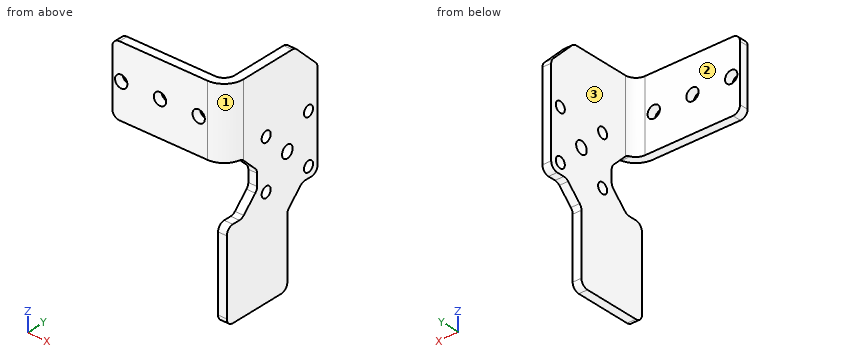
```python
from build123d import *

# Parameters (mm, degrees)
T_LE_DE_BASE_PLI_E1_DEPTH    = 40
BOSS_EXTRU_1_DEPTH           = 5
ENL_V_MAT_EXTRU_1_DEPTH      = 117.833214455
ENL_V_MAT_EXTRU_1_DEPTH_BACK = 117.833214455
ESQUISSE8_R                  = 3.5
ESQUISSE8_R_2                = 3
ESQUISSE10_W                 = 50
ESQUISSE10_H                 = 20
BOSS_EXTRU_2_DEPTH           = 5
ENL_V_MAT_EXTRU_2_DEPTH      = 117.833214455
ENL_V_MAT_EXTRU_2_DEPTH_BACK = 117.833214455
ESQUISSE9_R                  = 3.5
ENL_V_MAT_EXTRU_3_DEPTH      = 115.127122105
ENL_V_MAT_EXTRU_3_DEPTH_BACK = 115.127122105
ESQUISSE11_W                 = 50
ESQUISSE11_H                 = 20
CHANFREIN1_SIZE              = 10
CONG_1_R                     = 4


# Read off the part's stored shape, not the designer's step: Tôle de base pliée1
with BuildPart() as part:
    # Tôle de base pliée1 outline → Tôle de base pliée1 (new body)
    with BuildSketch(Plane.XY):
        with BuildLine():
            Line((65, 6), (65, 40))
            Line((65, 40), (60, 40))
            Line((60, 40), (60, 6))
            ThreePointArc((60, 6), (58.242640687, 1.757359313), (54, 0))
            Line((54, 0), (0, 0))
            Line((0, 0), (0, -5))
            Line((0, -5), (54, -5))
            ThreePointArc((54, -5), (61.778174593, -1.778174593), (65, 6))
        make_face()
    extrude(amount=T_LE_DE_BASE_PLI_E1_DEPTH)

    # Esquisse7 → Boss.-Extru.1 (add)
    with BuildSketch(Plane.ZY.offset(-60)):
        Polygon((25, 55), (-80, 55), (-80, 15), (0, 15), (40, 40), align=None)
    extrude(amount=-BOSS_EXTRU_1_DEPTH)

    # Esquisse8 → Enlèv. mat.-Extru.1 (cut, two sides: drawn at the far end of the back side and taken through both)
    with BuildSketch(Plane(origin=(65, 0, 0), x_dir=(0, 0, -1), z_dir=(1, 0, 0)).offset(-ENL_V_MAT_EXTRU_1_DEPTH_BACK)):
        with Locations(Location((10, 35, 0), (0, 0, 180))):
            Circle(ESQUISSE8_R)
        with Locations(Location((24, 49, 0), (0, 0, 180))):
            Circle(ESQUISSE8_R_2)
        with Locations(Location((24, 21, 0), (0, 0, 180))):
            Circle(ESQUISSE8_R_2)
        with Locations(Location((-4, 21, 0), (0, 0, 180))):
            Circle(ESQUISSE8_R_2)
        with Locations(Location((-4, 49, 0), (0, 0, 180))):
            Circle(ESQUISSE8_R_2)
    extrude(amount=ENL_V_MAT_EXTRU_1_DEPTH + ENL_V_MAT_EXTRU_1_DEPTH_BACK, mode=Mode.SUBTRACT)

    # Esquisse10 → Boss.-Extru.2 (add)
    with BuildSketch(Plane.ZY.offset(-60)):
        with Locations((-55, 5)):
            Rectangle(ESQUISSE10_W, ESQUISSE10_H)
    extrude(amount=-BOSS_EXTRU_2_DEPTH)

    # Esquisse9 → Enlèv. mat.-Extru.2 (cut, two sides: drawn at the far end of the back side and taken through both)
    with BuildSketch(Plane(origin=(0, 0, 0), x_dir=(1, 0, 0), z_dir=(0, 1, 0)).offset(-ENL_V_MAT_EXTRU_2_DEPTH_BACK)):
        with Locations(Location((5, -20, 0), (0, 0, 270))):
            Circle(ESQUISSE9_R)
        with Locations(Location((27, -20, 0), (0, 0, 270))):
            Circle(ESQUISSE9_R)
        with Locations(Location((49, -20, 0), (0, 0, 270))):
            Circle(ESQUISSE9_R)
    extrude(amount=ENL_V_MAT_EXTRU_2_DEPTH + ENL_V_MAT_EXTRU_2_DEPTH_BACK, mode=Mode.SUBTRACT)

    # Esquisse11 → Enlèv. mat.-Extru.3 (cut, two sides: drawn at the far end of the back side and taken through both)
    with BuildSketch(Plane.ZY.offset(-60).offset(-ENL_V_MAT_EXTRU_3_DEPTH_BACK)):
        with Locations((-55, 45)):
            Rectangle(ESQUISSE11_W, ESQUISSE11_H)
    extrude(amount=ENL_V_MAT_EXTRU_3_DEPTH + ENL_V_MAT_EXTRU_3_DEPTH_BACK, mode=Mode.SUBTRACT)

    # Chanfrein1
    chanfrein1_edges = [part.edges().sort_by_distance(p)[0] for p in [
        (62.5, 15, 0),
        (62.5, 15, -30),
        (62.5, 35, -30),
    ]]
    chamfer(chanfrein1_edges, length=CHANFREIN1_SIZE)

    # Congé1
    cong_1_edges = [part.edges().sort_by_distance(p)[0] for p in [
        (62.5, 55, -30),
        (62.5, 35, -80),
        (62.5, 35, -40),
        (62.5, 45, -30),
        (62.5, 5, -30),
        (62.5, 15, -10),
        (62.5, 15, -20),
        (62.435265467, 5, 0),
        (0, -2.5, 40),
        (62.5, 55, 25),
        (62.5, 40, 40),
        (0, -2.5, 0),
        (62.5, -5, -80),
        (62.5, -5, -30),
    ]]
    fillet(cong_1_edges, radius=CONG_1_R)


solid = part.part
```
Read the model definition and answer for the solid it produces. Units are mm, in the model's axes. Face numbers are marked on the shaded views. A direction names the side the tool comes from. Give positions to 0.01 mm unless a question says otherwise; leave off trailing zeros. Write each loop counter-clockwise with the first axis right and the second up, starting at its lowest first coordinate (ties: lowest second). Pieces come first, ordered by that corner, then holes. Notation, with made-up numbers: (53.25, 28.25) - (110.25, 28.25) arc R20 cw to (110.25, 67.25) - close; hole circle Ø9 at (3.25, 52.25). An arc over 180 degrees is marked (long way). Write item = value, one per line. Start each with the question number.
Item 1: Each of these flat-tipped pins is pushed along its axis until it touches: P1, Ø1.5, axis at x = 34, z = 28, coming from the +Y side; P2, Ø7, axis at y = 21, z = 4, coming from the -X side; P3, Ø3.5, axis at y = 49, z = 4, coming from the +X side; P4, Ø2, axis at x = 63.5, y = 48.5, coming from the -Z side. Where does it stop, or does it pass through?
Item 2: Find section B-B (y = 8). Give the vertices of the cut face in (x, z), then the cut area to 3 significant figures.
Item 3: A tool of negligible diameter and unlimited length cuts with its end or side. For the marked faces 1, 2 and 3, from which of +Z, -Z, +X, -X, +Y, -Y can it reach the whole face along a straight path? Write none if from no direction.
Item 4: Find section C-C (x = 49). Give the vertices of the cut face in (y, z), then the cut area to 3 significant figures.
Item 5: Find section A-A (y = 21). Give the vertices of the cut face in (x, z), then the cut area to 3 significant figures.
Item 6: Find section D-D (z = -24). Give the vertices of the cut face in (x, y), then the cut area to 3 significant figures.
Item 7: Find the intervals of material crossed by probe 1 along X at (y, z) = (-2, 20); probe 2 along Y at (x, z) = (61.2, 4); probe 3 along X at (y, z) = (-3.3, 20), in increasing order. Write a range as [from, to].
Response:
q1.P1 = 0
q1.P2 = 60
q1.P3 = through
q1.P4 = -30
q2.outline = (60, -80) - (65, -80) - (65, -27) - (60, -27) - close; (60, -3) - (65, -3) - (65, 40) - (60, 40) - close
q2.area = 480 mm²
q3.face_1 = +Z, +X, -Y
q3.face_2 = +Z, -Z, -X, +Y
q3.face_3 = -Z, -X, +Y
q4.outline = (-5, 0) - (0, 0) - (0, 16.5) - (-5, 16.5) - close; (-5, 23.5) - (0, 23.5) - (0, 40) - (-5, 40) - close
q4.area = 165 mm²
q5.outline = (60, -80) - (65, -80) - (65, -27) - (60, -27) - close; (60, -21) - (65, -21) - (65, 1) - (60, 1) - close; (60, 7) - (65, 7) - (65, 40) - (60, 40) - close
q5.area = 540 mm²
q6.outline = (60, 11) - (65, 11) - (65, 18) - (60, 18) - close; (60, 24) - (65, 24) - (65, 46) - (60, 46) - close; (60, 52) - (65, 52) - (65, 55) - (60, 55) - close
q6.area = 160 mm²
q7.probe_1 = [0, 1.5], [8.5, 23.5], [30.5, 45.5], [52.5, 61.55]
q7.probe_2 = [-2.32, 18], [24, 46], [52, 55]
q7.probe_3 = [0, 1.5], [8.5, 23.5], [30.5, 45.5], [52.5, 59.87]
